from build123d import *

# Parameters (mm, degrees)
F0_W     = 38.1
F0_H     = 63.5
F1_DEPTH = 104.775
F3_DEPTH = 38.101
F4_R     = 6.35
F5_DEPTH = 12.7
F6_R     = 3.175
F7_DEPTH = 50.801
F8_W     = 25.4
F8_H     = 19.05
F9_DEPTH = 38.101


with BuildPart() as f1:
    # F0 (on Right) → F1 (new body, symmetric)
    with BuildSketch(Plane.YZ):
        Rectangle(F0_W, F0_H)
    extrude(amount=F1_DEPTH, both=True)

    # F2 (on face) → F3 (cut, through all)
    with BuildSketch(Plane.XZ.offset(19.05)):
        with BuildLine():
            ThreePointArc((79.375, 0), (97.335512, -7.439488), (104.775, -25.4))
            Line((104.775, -25.4), (104.775, 31.75))
            Line((104.775, 31.75), (10.795, 31.75))
            ThreePointArc((10.795, 31.75), (21.571307, 27.286307), (26.035, 16.51))
            Line((26.035, 16.51), (26.035, 15.24))
            ThreePointArc((26.035, 15.24), (30.498693, 4.463693), (41.275, 0))
            Line((41.275, 0), (79.375, 0))
        make_face()
    extrude(amount=-F3_DEPTH, mode=Mode.SUBTRACT)

    # F4 (on face) → F5 (cut)
    with BuildSketch(Plane(origin=(0, 0, -31.75), x_dir=(1, 0, 0), z_dir=(0, 0, -1))):
        with Locations((-85.725, 0)):
            Circle(F4_R)
        with Locations((-15.875, 0)):
            Circle(F4_R)
    extrude(amount=-F5_DEPTH, mode=Mode.SUBTRACT)

    # F6 (on face) → F7 (cut, through all)
    with BuildSketch(Plane(origin=(0, 0, -19.05), x_dir=(1, 0, 0), z_dir=(0, 0, -1))):
        with Locations((-85.725, 0)):
            Circle(F6_R)
        with Locations((-15.875, 0)):
            Circle(F6_R)
    extrude(amount=-F7_DEPTH, mode=Mode.SUBTRACT)

    # F8 (on face) → F9 (cut, through all)
    with BuildSketch(Plane.XZ.offset(19.05)):
        with Locations((-47.625, 22.225)):
            Rectangle(F8_W, F8_H)
    extrude(amount=-F9_DEPTH, mode=Mode.SUBTRACT)


solid = f1.part
Verification items for the finished model (mm, model axes). A direction names the side the tool comes from. Give positions to 0.01 mm unless a question says otherwise; leave off trailing zeros. Loops run counter-clockwise (first coordinate to the right, second up) from the corner with the lowest first, then second, coordinate; pieces in that order, holes last.
1. Go/stop test with flat-tipped pins: P1, Ø4, axis at y = 14, z = 13, coming from the +X side; P2, Ø0.6, axis at y = -3, z = 16, coming from the +X side (3 decimals); P3, Ø10, axis at x = -15.875, y = 0, coming from the -Z side. Record where each tip stops, or that it passes through.
Derived:
P1: stops at x = 26.64
P2: stops at x = 26.035
P3: stops at z = -19.05
2. Cross-section at D-D on y = -10.5. Record the cut outline in (x, z) (3 decimals).
Derived:
outline: (-104.775, -31.75) - (104.775, -31.75) - (104.775, -25.4) arc R25.4 ccw to (79.375, 0) - (41.275, 0) arc R15.24 cw to (26.035, 15.24) - (26.035, 16.51) arc R15.24 ccw to (10.795, 31.75) - (-34.925, 31.75) - (-34.925, 12.7) - (-60.325, 12.7) - (-60.325, 31.75) - (-104.775, 31.75) - close
3. Cross-section at C-C on z = -9.5. Record the cut outline in (x, y) (3 decimals), and give its area (3 significant figures).
Derived:
outline: (-104.775, -19.05) - (99.183, -19.05) - (99.183, 19.05) - (-104.775, 19.05) - close; hole circle Ø6.35 at (-85.725, 0); hole circle Ø6.35 at (-15.875, 0)
area: 7,710 mm2
4. Cross-section at B-B on x = -86.5. Record the cut outline in (y, z).
Derived:
outline: (-19.05, -31.75) - (-6.3, -31.75) - (-6.3, -19.05) - (-3.08, -19.05) - (-3.08, 31.75) - (-19.05, 31.75) - close; (3.08, -19.05) - (6.3, -19.05) - (6.3, -31.75) - (19.05, -31.75) - (19.05, 31.75) - (3.08, 31.75) - close
5. Cross-section at A-A on y = 0. Count the separate pieces of the cut face and the enclosed holes in it, and give its area (3 significant figures).
Derived:
separate pieces: 3
enclosed holes: 0
area: 9,220 mm2
6. Tool access check on faces 4 (the cylindrical face through (-20.914, 3.864, -25.489)), 5 (the flat face through (60, 0, 0)), 6 (the flat face through (-48, 0, 12.7)). Record the directions out of +Z, -Z, +X, -X, +Y, -Y that give a thin tool (end or side, any length) a straight path to the whole face; none if there is none.
Derived:
face 4: -Z
face 5: +Z, +X, +Y, -Y
face 6: +Z, +Y, -Y
7. Release check for a two-part mould opening along X. For faces 1 (the flat face through (1, 0, -31.75)), 2 (the flat face through (104.775, 0, -29)), 3 (the cylindrical face through (-92.07, -0.28, -25.49)) record: +X half, -X half, draft (parallel to the pull), parting line (faces both ways), or undercut.
Derived:
face 1: draft
face 2: +X half
face 3: undercut
8. Material ranges on probe 1 along X at (y, z) = (0, -25.5) (3 decimals); probe 2 along X at (y, z) = (0, 22) (3 decimals); probe 3 along X at (y, z) = (0, 11) (3 decimals), recorded low to high.
Derived:
probe 1: x = -104.775 to -92.075, -79.375 to -22.225, -9.525 to 104.775
probe 2: x = -104.775 to -88.9, -82.55 to -60.325, -34.925 to -19.05, -12.7 to 25.012
probe 3: x = -104.775 to -88.9, -82.55 to -19.05, -12.7 to 26.637
